from build123d import *

# Parameters (mm, degrees)
SKETCH1_W           = 60
SKETCH1_H           = 41
BOSS_EXTRUDE1_DEPTH = 2
SKETCH2_R           = 9
CUT_EXTRUDE2_DEPTH  = 1
CUT_EXTRUDE3_DEPTH  = 1
SKETCH4_W           = 8
SKETCH4_H           = 8
CUT_EXTRUDE4_DEPTH  = 1
BOSS_EXTRUDE2_START = 58
BOSS_EXTRUDE2_DEPTH = 58
SKETCH6_R           = 1.6
CUT_EXTRUDE5_DEPTH  = 18
CHAMFER2_SIZE       = 0.5
CHAMFER3_SIZE       = 1
SKETCH7_R           = 1.6
CUT_EXTRUDE6_DEPTH  = 93.978492137
FILLET1_R           = 2
BOSS_EXTRUDE3_DEPTH = 2.6
SKETCH11_W          = 2.5
SKETCH11_H          = 1
BOSS_EXTRUDE4_DEPTH = 54
FILLET2_R           = 2


with BuildPart() as part:
    # Sketch1 → Boss-Extrude1 (new body)
    with BuildSketch(Plane(origin=(0, 0, 0), x_dir=(1, 0, 0), z_dir=(0, 1, 0))):
        with Locations((-30, 20.5)):
            Rectangle(SKETCH1_W, SKETCH1_H)
    extrude(amount=BOSS_EXTRUDE1_DEPTH)

    # Sketch2 → Cut-Extrude2 (cut)
    with BuildSketch(Plane(origin=(0, 2, 0), x_dir=(1, 0, 0), z_dir=(0, 1, 0))):
        with Locations(Location((-49, 11, 0), (0, 0, 270))):
            Circle(SKETCH2_R)
        with Locations(Location((-30, 11, 0), (0, 0, 270))):
            Circle(SKETCH2_R)
        with Locations(Location((-11, 11, 0), (0, 0, 270))):
            Circle(SKETCH2_R)
        with Locations(Location((-30, 30, 0), (0, 0, 270))):
            Circle(SKETCH2_R)
        with Locations(Location((-11, 30, 0), (0, 0, 270))):
            Circle(SKETCH2_R)
        with Locations(Location((-49, 30, 0), (0, 0, 270))):
            Circle(SKETCH2_R)
    extrude(amount=-CUT_EXTRUDE2_DEPTH, mode=Mode.SUBTRACT)

    # Sketch3 → Cut-Extrude3 (cut)
    with BuildSketch(Plane.XZ):
        with BuildLine():
            Line((-5.5, -35.497915762), (-5.5, -5.497915762))
            ThreePointArc((-5.5, -5.497915762), (-11, -1.895831523), (-16.5, -5.497915762))
            Line((-16.5, -5.497915762), (-16.5, -35.497915762))
            ThreePointArc((-16.5, -35.497915762), (-11, -39.1), (-5.5, -35.497915762))
        make_face()
        with BuildLine():
            Line((-35.5, -35.497915762), (-35.5, -5.497915762))
            ThreePointArc((-35.5, -5.497915762), (-30, -1.895831523), (-24.5, -5.497915762))
            Line((-24.5, -5.497915762), (-24.5, -35.497915762))
            ThreePointArc((-24.5, -35.497915762), (-30, -39.1), (-35.5, -35.497915762))
        make_face()
        with BuildLine():
            Line((-54.5, -35.497915762), (-54.5, -5.497915762))
            ThreePointArc((-54.5, -5.497915762), (-49, -1.895831523), (-43.5, -5.497915762))
            Line((-43.5, -5.497915762), (-43.5, -35.497915762))
            ThreePointArc((-43.5, -35.497915762), (-49, -39.1), (-54.5, -35.497915762))
        make_face()
    extrude(amount=-CUT_EXTRUDE3_DEPTH, mode=Mode.SUBTRACT)

    # Sketch4 → Cut-Extrude4 (cut)
    with BuildSketch(Plane.XZ):
        with Locations((-20.5, -20.501096576)):
            Rectangle(SKETCH4_W, SKETCH4_H)
    extrude(amount=-CUT_EXTRUDE4_DEPTH, mode=Mode.SUBTRACT)

    # Sketch5 → Boss-Extrude2 (add)
    with BuildSketch(Plane(origin=(0, 2, 0), x_dir=(1, 0, 0), z_dir=(0, 1, 0)).offset(BOSS_EXTRUDE2_START)):
        with BuildLine():
            Line((-20, 30), (-21, 30))
            ThreePointArc((-21, 30), (-23.636038969, 23.636038969), (-30, 21))
            ThreePointArc((-30, 21), (-36.363961031, 23.636038969), (-39, 30))
            Line((-39, 30), (-40, 30))
            ThreePointArc((-40, 30), (-42.636038969, 23.636038969), (-49, 21))
            Line((-49, 21), (-49, 20))
            ThreePointArc((-49, 20), (-42.636038969, 17.363961031), (-40, 11))
            Line((-40, 11), (-39, 11))
            ThreePointArc((-39, 11), (-36.363961031, 17.363961031), (-30, 20))
            ThreePointArc((-30, 20), (-23.636038969, 17.363961031), (-21, 11))
            Line((-21, 11), (-20, 11))
            ThreePointArc((-20, 11), (-17.363961031, 17.363961031), (-11, 20))
            Line((-11, 20), (-11, 21))
            ThreePointArc((-11, 21), (-17.363961031, 23.636038969), (-20, 30))
        make_face()
        with BuildLine():
            Line((-58, 30), (-60, 30))
            Line((-60, 30), (-60, 41))
            Line((-60, 41), (-49, 41))
            Line((-49, 41), (-49, 39))
            ThreePointArc((-49, 39), (-55.363961031, 36.363961031), (-58, 30))
        make_face()
        with BuildLine():
            Line((-58, 11), (-60, 11))
            Line((-60, 11), (-60, 0))
            Line((-60, 0), (-49, 0))
            Line((-49, 0), (-49, 2))
            ThreePointArc((-49, 2), (-55.363961031, 4.636038969), (-58, 11))
        make_face()
        with BuildLine():
            Line((-2, 11), (0, 11))
            Line((0, 11), (0, 0))
            Line((0, 0), (-11, 0))
            Line((-11, 0), (-11, 2))
            ThreePointArc((-11, 2), (-4.636038969, 4.636038969), (-2, 11))
        make_face()
        with BuildLine():
            Line((-2, 30), (0, 30))
            Line((0, 30), (0, 41))
            Line((0, 41), (-11, 41))
            Line((-11, 41), (-11, 39))
            ThreePointArc((-11, 39), (-4.636038969, 36.363961031), (-2, 30))
        make_face()
    extrude(amount=-BOSS_EXTRUDE2_DEPTH)

    # Sketch6 → Cut-Extrude5 (cut)
    with BuildSketch(Plane(origin=(0, 60, 0), x_dir=(1, 0, 0), z_dir=(0, 1, 0))):
        with Locations(Location((-20.5, 20.5, 0), (0, 0, 270))):
            Circle(SKETCH6_R)
        with Locations(Location((-39.5, 20.5, 0), (0, 0, 270))):
            Circle(SKETCH6_R)
        with Locations(Location((-57.25, 2.75, 0), (0, 0, 270))):
            Circle(SKETCH6_R)
        with Locations(Location((-57.25, 38.25, 0), (0, 0, 270))):
            Circle(SKETCH6_R)
        with Locations(Location((-2.75, 2.75, 0), (0, 0, 270))):
            Circle(SKETCH6_R)
        with Locations(Location((-2.75, 38.25, 0), (0, 0, 270))):
            Circle(SKETCH6_R)
    extrude(amount=-CUT_EXTRUDE5_DEPTH, mode=Mode.SUBTRACT)

    # Chamfer2
    # the kernel refuses this chamfer: 0.5 mm, written as the material it takes off along each edge
    with BuildSketch(Plane(origin=(-40, 61.324152825, -11), x_dir=(1, 0, 0), z_dir=(0, -1, 0)), Plane(origin=(-21, 61.324152825, -11), x_dir=(1, 0, 0), z_dir=(0, -1, 0)), Plane(origin=(-49, 61.324152825, -21), x_dir=(0, 0, 1), z_dir=(0, -1, 0)), Plane(origin=(-39, 61.324152825, -30), x_dir=(-1, 0, 0), z_dir=(0, -1, 0)), Plane(origin=(-20, 61.324152825, -30), x_dir=(-1, 0, 0), z_dir=(0, -1, 0)), Plane(origin=(-11, 61.324152825, -20), x_dir=(0, 0, -1), z_dir=(0, -1, 0))) as chamfer2_piece_1:
        with BuildLine():
            Line((CHAMFER2_SIZE, 0), (-0.014731413, -0.514731413))
            ThreePointArc((-0.014731413, -0.514731413), (-0.003894786, -0.264747015), (0, 0))
            Line((0, 0), (CHAMFER2_SIZE, 0))
        make_face()
    extrude(amount=59.324152825, mode=Mode.SUBTRACT)
    with BuildSketch(Plane(origin=(-39, 61.324152825, -11), x_dir=(-1, 0, 0), z_dir=(0, -1, 0)), Plane(origin=(-20, 61.324152825, -11), x_dir=(-1, 0, 0), z_dir=(0, -1, 0)), Plane(origin=(-40, 61.324152825, -30), x_dir=(1, 0, 0), z_dir=(0, -1, 0)), Plane(origin=(-21, 61.324152825, -30), x_dir=(1, 0, 0), z_dir=(0, -1, 0)), Plane(origin=(-11, 61.324152825, -21), x_dir=(0, 0, 1), z_dir=(0, -1, 0))) as chamfer2_piece_2:
        with BuildLine():
            Line((CHAMFER2_SIZE, 0), (-0.014731413, 0.514731413))
            ThreePointArc((-0.014731413, 0.514731413), (-0.003894786, 0.264747015), (0, 0))
            Line((0, 0), (CHAMFER2_SIZE, 0))
        make_face()
    extrude(amount=59.324152825, mode=Mode.SUBTRACT)
    with BuildSketch(Plane(origin=(-49, 61.324152825, -20), x_dir=(0.999590710311118, 0, 0.02860789855467639), z_dir=(0, -1, 0))) as chamfer2_piece_3:
        with BuildLine():
            Line((0.514942174, 0), (-CHAMFER2_SIZE * 0.0286078985547, -CHAMFER2_SIZE * 0.999590710311))
            Line((-CHAMFER2_SIZE * 0.0286078985547, -CHAMFER2_SIZE * 0.999590710311), (0, 0))
            ThreePointArc((0, 0), (0.264750079, -0.003680664), (0.514942174, 0))
        make_face()
    extrude(amount=59.324152825, mode=Mode.SUBTRACT)

    # Chamfer3
    # the kernel refuses this chamfer: 1 mm, written as the material it takes off along each edge
    with BuildSketch(Plane(origin=(-2, 62.73772815, -30), x_dir=(1, 0, 0), z_dir=(0, -1, 0)), Plane(origin=(-49, 62.73772815, -39), x_dir=(0, 0, -1), z_dir=(0, -1, 0)), Plane(origin=(-11, 62.73772815, -2), x_dir=(0, 0, 1), z_dir=(0, -1, 0))) as chamfer3_piece_1:
        with BuildLine():
            Line((CHAMFER3_SIZE, 0), (-0.062996063, -1.062996063))
            ThreePointArc((-0.062996063, -1.062996063), (-0.016662827, -0.547405922), (0, 0))
            Line((0, 0), (CHAMFER3_SIZE, 0))
        make_face()
    extrude(amount=60.73772815, mode=Mode.SUBTRACT)
    with BuildSketch(Plane(origin=(0, 62.571682988, -30), x_dir=(0, 0, -1), z_dir=(0, -1, 0)), Plane(origin=(-49, 62.571682988, -41), x_dir=(-1, 0, 0), z_dir=(0, -1, 0)), Plane(origin=(-60, 62.571682988, -11), x_dir=(0, 0, 1), z_dir=(0, -1, 0)), Plane(origin=(-11, 62.571682988, 0), x_dir=(1, 0, 0), z_dir=(0, -1, 0))) as chamfer3_piece_2:
        Polygon((CHAMFER3_SIZE, 0), (0, -CHAMFER3_SIZE), (0, 0), align=None)
    extrude(amount=60.571682988, mode=Mode.SUBTRACT)
    with BuildSketch(Plane(origin=(-11, 62.73772815, -39), x_dir=(0, 0, -1), z_dir=(0, -1, 0)), Plane(origin=(-58, 62.73772815, -30), x_dir=(-1, 0, 0), z_dir=(0, -1, 0)), Plane(origin=(-49, 62.73772815, -2), x_dir=(0, 0, 1), z_dir=(0, -1, 0)), Plane(origin=(-2, 62.73772815, -11), x_dir=(1, 0, 0), z_dir=(0, -1, 0))) as chamfer3_piece_3:
        with BuildLine():
            Line((CHAMFER3_SIZE, 0), (-0.062996063, 1.062996063))
            ThreePointArc((-0.062996063, 1.062996063), (-0.016662827, 0.547405922), (0, 0))
            Line((0, 0), (CHAMFER3_SIZE, 0))
        make_face()
    extrude(amount=60.73772815, mode=Mode.SUBTRACT)
    with BuildSketch(Plane(origin=(-11, 62.571682988, -41), x_dir=(1, 0, 0), z_dir=(0, -1, 0)), Plane(origin=(-60, 62.571682988, -30), x_dir=(0, 0, -1), z_dir=(0, -1, 0)), Plane(origin=(-49, 62.571682988, 0), x_dir=(-1, 0, 0), z_dir=(0, -1, 0)), Plane(origin=(0, 62.571682988, -11), x_dir=(0, 0, 1), z_dir=(0, -1, 0))) as chamfer3_piece_4:
        Polygon((CHAMFER3_SIZE, 0), (0, CHAMFER3_SIZE), (0, 0), align=None)
    extrude(amount=60.571682988, mode=Mode.SUBTRACT)
    with BuildSketch(Plane(origin=(-58, 62.73772815, -11), x_dir=(0.05915894925917608, 0, 0.9982485756175915), z_dir=(0, -1, 0))) as chamfer3_piece_5:
        with BuildLine():
            Line((1.064861087, 0), (-CHAMFER3_SIZE * 0.0591589492592, CHAMFER3_SIZE * 0.998248575618))
            Line((-CHAMFER3_SIZE * 0.0591589492592, CHAMFER3_SIZE * 0.998248575618), (0, 0))
            ThreePointArc((0, 0), (0.547432937, 0.015750315), (1.064861087, 0))
        make_face()
    extrude(amount=60.73772815, mode=Mode.SUBTRACT)

    # Sketch7 → Cut-Extrude6 (cut, through all)
    with BuildSketch(Plane(origin=(0, 2, 0), x_dir=(1, 0, 0), z_dir=(0, 1, 0))):
        with Locations(Location((-57.5, 20.5, 0), (0, 0, 270))):
            Circle(SKETCH7_R)
        with Locations(Location((-2.5, 20.5, 0), (0, 0, 270))):
            Circle(SKETCH7_R)
    extrude(amount=-CUT_EXTRUDE6_DEPTH, mode=Mode.SUBTRACT)

    # Fillet1
    # the kernel refuses this fillet: 2 mm, written as the material it takes off along each edge
    with BuildSketch(Plane(origin=(-16.5, -5, -16.501096576), x_dir=(0, 0, 1), z_dir=(0, 1, 0)), Plane(origin=(-24.5, -5, -16.501096576), x_dir=(1, 0, 0), z_dir=(0, 1, 0))) as fillet1_piece_1:
        with BuildLine():
            CenterArc((FILLET1_R, -FILLET1_R), FILLET1_R, 90, 90)
            Line((0, -FILLET1_R), (0, 0))
            Line((0, 0), (FILLET1_R, 0))
        make_face()
    extrude(amount=6, mode=Mode.SUBTRACT)
    with BuildSketch(Plane(origin=(-16.5, -5, -24.501096576), x_dir=(0, 0, -1), z_dir=(0, 1, 0)), Plane(origin=(-24.5, -5, -24.501096576), x_dir=(1, 0, 0), z_dir=(0, 1, 0))) as fillet1_piece_2:
        with BuildLine():
            CenterArc((FILLET1_R, FILLET1_R), FILLET1_R, 180, 90)
            Line((0, FILLET1_R), (0, 0))
            Line((0, 0), (FILLET1_R, 0))
        make_face()
    extrude(amount=6, mode=Mode.SUBTRACT)
    with BuildSketch(Plane(origin=(0, -5, 0), x_dir=(-1, 0, 0), z_dir=(0, 1, 0)), Plane(origin=(-60, 65, 0), x_dir=(1, 0, 0), z_dir=(0, -1, 0)), Plane(origin=(-60, 65, -41), x_dir=(0, 0, 1), z_dir=(0, -1, 0)), Plane(origin=(0, -5, -41), x_dir=(0, 0, 1), z_dir=(0, 1, 0))) as fillet1_piece_3:
        with BuildLine():
            CenterArc((FILLET1_R, -FILLET1_R), FILLET1_R, 90, 90)
            Line((0, -FILLET1_R), (0, 0))
            Line((0, 0), (FILLET1_R, 0))
        make_face()
    extrude(amount=70, mode=Mode.SUBTRACT)

    # Sketch9 → Boss-Extrude3 (add)
    with BuildSketch(Plane(origin=(0, 0, -41), x_dir=(-1, 0, 0), z_dir=(0, 0, -1))):
        Polygon((52.5, 0), (54.5, 0), (54.5, 56), (52.5, 56), (52.5, 2), (50, 2), (50, 0), align=None)
        Polygon((5.5, 0), (7.5, 0), (10, 0), (10, 2), (7.5, 2), (7.5, 56), (5.5, 56), align=None)
    extrude(amount=BOSS_EXTRUDE3_DEPTH)

    # Sketch11 → Boss-Extrude4 (add)
    with BuildSketch(Plane(origin=(0, 2, 0), x_dir=(1, 0, 0), z_dir=(0, 1, 0))):
        with Locations((-8.75, 43.1)):
            Rectangle(SKETCH11_W, SKETCH11_H)
        with Locations((-51.25, 43.1)):
            Rectangle(SKETCH11_W, SKETCH11_H)
    extrude(amount=BOSS_EXTRUDE4_DEPTH)

    # Fillet2
    fillet2_edges = [part.edges().sort_by_distance(p)[0] for p in [
        (-54.5, 28, -43.6),
        (-5.5, 28, -43.6),
    ]]
    fillet(fillet2_edges, radius=FILLET2_R)


solid = part.part
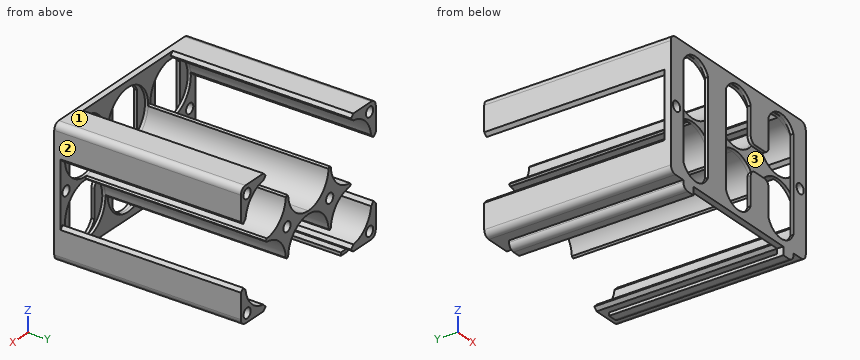
Work out the finished part from the listing and answer in its coordinate system (mm). Face numbers are marked on the shaded views. Give positions to 0.01 mm unless a question says otherwise; leave off trailing zeros. Loops run counter-clockwise (first coordinate to the right, second up) from the corner with the lowest first, then second, coordinate; pieces in that order, holes last. Notation, with made-up numbers: (25, -34.5) - (64, -34.5) arc R13 cw to (64, -28.5) - close; hole circle Ø3 at (6.5, -20.5). An arc over 180 degrees is marked (long way). Answer in a Markdown table with one row per item. Add a question column.
Q1. Consider line 1 along X through (y, z) = (1.05, -20.5); line 2 along X through (y, z) = (47, -10); line 3 along X through (y, z) = (44, -38). Determine where each line is inside the solid, lowest interval first.
Q2. Each of these flat-tipped pins is pushed along its axis until it touches: P1, Ø2, axis at x = -17.5, z = -30, coming from the +Y side; P2, Ø6, axis at x = -53.5, z = -21.5, coming from the +Y side; P3, Ø3, axis at x = -20.5, y = 15.5, coming from the +Z side. Where does it stop, or does it pass through?
Q3. Determine the mould class of the marked faces 1, 2 and 3 for opening direction Z: released by +Z, released by -Z, zero draft, split by the parting line, or undercut.
Q4. The part is cut by section A-A (y = 54). State how many separate pieces and enclosed holes the cut face has, and give its area (3 significant figures).
Q5. The part is cut by section C-C (x = -36.5). Determine the outline of the cut face in (y, z).
Solution:
| question | item | result |
|---|---|---|
| 1 | line 1 | x = -60 to -59.1, -55.9 to -4.1, -0.9 to 0 |
| 1 | line 2 | x = -60 to -58, -2 to 0 |
| 1 | line 3 | x = -60 to -58.83, -55.67 to -53.12, -6.88 to -4.33, -1.17 to 0 |
| 2 | P1 | stops at y = 1 |
| 2 | P2 | stops at y = 2 |
| 2 | P3 | stops at z = -11 |
| 3 | face 1 | released by +Z |
| 3 | face 2 | zero draft |
| 3 | face 3 | undercut |
| 4 | separate pieces | 5 |
| 4 | enclosed holes | 6 |
| 4 | area | 395 mm² |
| 5 | outline | (0, -41) - (2, -41) - (2, -36.22) - (1, -36.22) - (1, -23.78) - (60, -23.78) - (60, -17.22) - (1, -17.22) - (1, -4.78) - (2, -4.78) - (2, 0) - (0, 0) - close |
